Could you check a few things on this model? Use its own coordinates, in mm. A direction names the side the tool comes from. Round coordinates to 2 decimals unless told otherwise and drop trailing zeros. Answer in a Markdown table with one row per item.
from build123d import *

# Parameters (mm, degrees)
SKETCH_1_R      = 2.5
EXTRUDE_1_DEPTH = 250


with BuildPart() as part:
    # 草图1 → 凸台-拉伸1 (new body)
    with BuildSketch(Plane.XY):
        with BuildLine():
            Line((3.9, 0), (3.9, 1.971572875))
            ThreePointArc((3.9, 1.971572875), (4.052240935, 2.73693974), (4.485786438, 3.385786438))
            Line((4.485786438, 3.385786438), (6.6, 5.5))
            Line((6.6, 5.5), (8.2, 5.5))
            Line((8.2, 5.5), (8.2, 3.1))
            Line((8.2, 3.1), (9.5, 3.1))
            ThreePointArc((9.5, 3.1), (9.853553391, 3.246446609), (10, 3.6))
            Line((10, 3.6), (10, 8.5))
            ThreePointArc((10, 8.5), (9.560660172, 9.560660172), (8.5, 10))
            Line((8.5, 10), (3.6, 10))
            ThreePointArc((3.6, 10), (3.246446609, 9.853553391), (3.1, 9.5))
            Line((3.1, 9.5), (3.1, 8.2))
            Line((3.1, 8.2), (5.5, 8.2))
            Line((5.5, 8.2), (5.5, 6.6))
            Line((5.5, 6.6), (3.385786438, 4.485786438))
            ThreePointArc((3.385786438, 4.485786438), (2.73693974, 4.052240935), (1.971572875, 3.9))
            Line((1.971572875, 3.9), (0, 3.9))
            Line((0, 3.9), (-1.971572875, 3.9))
            ThreePointArc((-1.971572875, 3.9), (-2.73693974, 4.052240935), (-3.385786438, 4.485786438))
            Line((-3.385786438, 4.485786438), (-5.5, 6.6))
            Line((-5.5, 6.6), (-5.5, 8.2))
            Line((-5.5, 8.2), (-3.1, 8.2))
            Line((-3.1, 8.2), (-3.1, 9.5))
            ThreePointArc((-3.1, 9.5), (-3.246446609, 9.853553391), (-3.6, 10))
            Line((-3.6, 10), (-8.5, 10))
            ThreePointArc((-8.5, 10), (-9.560660172, 9.560660172), (-10, 8.5))
            Line((-10, 8.5), (-10, 3.6))
            ThreePointArc((-10, 3.6), (-9.853553391, 3.246446609), (-9.5, 3.1))
            Line((-9.5, 3.1), (-8.2, 3.1))
            Line((-8.2, 3.1), (-8.2, 5.5))
            Line((-8.2, 5.5), (-6.6, 5.5))
            Line((-6.6, 5.5), (-4.485786438, 3.385786438))
            ThreePointArc((-4.485786438, 3.385786438), (-4.052240935, 2.73693974), (-3.9, 1.971572875))
            Line((-3.9, 1.971572875), (-3.9, 0))
            Line((-3.9, 0), (-3.9, -1.971572875))
            ThreePointArc((-3.9, -1.971572875), (-4.052240935, -2.73693974), (-4.485786438, -3.385786438))
            Line((-4.485786438, -3.385786438), (-6.6, -5.5))
            Line((-6.6, -5.5), (-8.2, -5.5))
            Line((-8.2, -5.5), (-8.2, -3.1))
            Line((-8.2, -3.1), (-9.5, -3.1))
            ThreePointArc((-9.5, -3.1), (-9.853553391, -3.246446609), (-10, -3.6))
            Line((-10, -3.6), (-10, -8.5))
            ThreePointArc((-10, -8.5), (-9.560660172, -9.560660172), (-8.5, -10))
            Line((-8.5, -10), (-3.6, -10))
            ThreePointArc((-3.6, -10), (-3.246446609, -9.853553391), (-3.1, -9.5))
            Line((-3.1, -9.5), (-3.1, -8.2))
            Line((-3.1, -8.2), (-5.5, -8.2))
            Line((-5.5, -8.2), (-5.5, -6.6))
            Line((-5.5, -6.6), (-3.385786438, -4.485786438))
            ThreePointArc((-3.385786438, -4.485786438), (-2.73693974, -4.052240935), (-1.971572875, -3.9))
            Line((-1.971572875, -3.9), (0, -3.9))
            Line((0, -3.9), (1.971572875, -3.9))
            ThreePointArc((1.971572875, -3.9), (2.73693974, -4.052240935), (3.385786438, -4.485786438))
            Line((3.385786438, -4.485786438), (5.5, -6.6))
            Line((5.5, -6.6), (5.5, -8.2))
            Line((5.5, -8.2), (3.1, -8.2))
            Line((3.1, -8.2), (3.1, -9.5))
            ThreePointArc((3.1, -9.5), (3.246446609, -9.853553391), (3.6, -10))
            Line((3.6, -10), (8.5, -10))
            ThreePointArc((8.5, -10), (9.560660172, -9.560660172), (10, -8.5))
            Line((10, -8.5), (10, -3.6))
            ThreePointArc((10, -3.6), (9.853553391, -3.246446609), (9.5, -3.1))
            Line((9.5, -3.1), (8.2, -3.1))
            Line((8.2, -3.1), (8.2, -5.5))
            Line((8.2, -5.5), (6.6, -5.5))
            Line((6.6, -5.5), (4.485786438, -3.385786438))
            ThreePointArc((4.485786438, -3.385786438), (4.052240935, -2.73693974), (3.9, -1.971572875))
            Line((3.9, -1.971572875), (3.9, 0))
        make_face()
        Circle(SKETCH_1_R, mode=Mode.SUBTRACT)
    extrude(amount=EXTRUDE_1_DEPTH)


solid = part.part
1) For faces 4 (the face through (-3.9, 0, 123)), 5 (the face through (0, 3.9, 123)), 6 (the face through (0, -3.9, 123)), which set-ups out of +Z, -Z, +X, -X, +Y, -Y let a thin tool reach every point of the face, with its end or its side?
Findings:
| item | result |
|---|---|
| face 4 | +Z, -Z, -X |
| face 5 | +Z, -Z, +Y |
| face 6 | +Z, -Z, -Y |
2) For pin 1 (5 mm diameter, centred on x = 0, y = -6.5, fed in from +Z); pin 2 (1.2 mm diameter, centred on x = 0, z = 141.5, fed in from -Y); pin 3 (0.7 mm diameter, centred on y = -9, z = 154.5, fed in from -X); pin 4 (1.2 mm diameter, centred on y = 0.5, z = 82.5, fed in from -X), each with a flat end and sliding along its axis, tell me the tip position at first contact or that it passes through.
Findings:
| item | result |
|---|---|
| pin 1 | passes through |
| pin 2 | stops at y = -3.9 |
| pin 3 | stops at x = -9.99 |
| pin 4 | stops at x = -3.9 |
3) Please list where these lines run through material, in increasing order: line 1 (Y direction, x = -8, z = 54.5); line 2 (Y direction, x = -3.5, z = 154); line 3 (Y direction, x = 0, z = 78).
Findings:
| item | result |
|---|---|
| line 1 | y = -10 to -5.5, 5.5 to 10 |
| line 2 | y = -9.99 to -8.2, -4.6 to 4.6, 8.2 to 9.99 |
| line 3 | y = -3.9 to -2.5, 2.5 to 3.9 |
4) Thinking about a two-plate mould opening in Y: for faces 1 (the face through (10, 6, 123)), 2 (the face through (6, -10, 123)), 3 (the face through (3.9, 0, 123)), which applies, +Y half, -Y half, draft (parallel to the pull), parting line (faces both ways), or undercut?
Findings:
| item | result |
|---|---|
| face 1 | draft |
| face 2 | -Y half |
| face 3 | undercut |
